The model under review builds one solid part; all positions refer to its coordinate system, in mm. Face numbers are marked on the shaded views. A direction names the side the tool comes from. Give positions to 0.01 mm unless a question says otherwise; leave off trailing zeros. Order: outer loops, then holes, each group sorted by start corner. A loop starts at its lowest first (then second) coordinate and runs counter-clockwise, first axis right, second up. Notation, with made-up numbers: (57, -29) - (68, -29) arc R21 ccw to (68, 7) - close; hole circle Ø3 at (49, 41). An arc over 180 degrees is marked (long way). Use CSV: the item, a comma, the result in double quotes. Start each with the question number.
1. Take a section at D-D, the plane x = 6. State the section outline as (y, z) points.
2. Take a section at B-B, the plane x = 43. State the section outline as (y, z) points.
3. Draft analysis for pull direction X (two halves, no side actions). For the marked faces 4, 5 and 6, state which applies: released by +X, released by -X, zero draft, split by the parting line, or undercut.
4. For pin 1 (6 mm diameter, centred on y = -4.5, z = -0.5, fed in from +X); pin 2 (2 mm diameter, centred on x = 15, y = -4.5, fed in from -Z); pin 3 (2 mm diameter, centred on y = -5, z = -4.5, fed in from -X), all flat-tipped, find the tip position at first contact; note any pin that passes through.
5. Take a section at A-A, the plane y = -3.25. State the section outline as (x, z) points.
6. Take a section at C-C, the plane y = 1.5. State the section outline as (x, z) points.
7. To check wall thickness, follow line 1 (Y direction, x = 36.5, z = -4.5); line 2 (X direction, y = 3, z = -2.25); line 3 (X direction, y = -1.75, z = -0.75). State the ranges of each line that lie inside material, in increasing order. Write a range as [from, to].
8. Machinability: for the marked faces 1, 2 and 3, which of the approach directions +Z, -Z, +X, -X, +Y, -Y give a long, thin tool a straight path to every point of the face, cutting with its end or side? Answer none if there is none.
```python
from build123d import *

# Parameters (mm, degrees)
BOSS_EXTRUDE1_DEPTH = 4
BOSS_EXTRUDE3_DEPTH = 2
BOSS_EXTRUDE4_DEPTH = 4
BOSS_EXTRUDE5_DEPTH = 2
BOSS_EXTRUDE6_DEPTH = 4


with BuildPart() as part:
    # Sketch1 → Boss-Extrude1 (new body)
    with BuildSketch(Plane(origin=(0, 0, 0), x_dir=(1, 0, 0), z_dir=(0, 1, 0))):
        with BuildLine():
            Line((-14.545827973, 6.554746402), (-17.81521366, 1.88557975))
            Line((-17.81521366, 1.88557975), (-10.442845262, -3.276608177))
            Line((-10.442845262, -3.276608177), (-8.148539516, -4))
            Line((-8.148539516, -4), (41.019227437, -1.767766953))
            Line((41.019227437, -1.767766953), (39.551460484, -0.3))
            Line((39.551460484, -0.3), (39.551460484, 4.117528082))
            ThreePointArc((39.551460484, 4.117528082), (40.137246921, 5.114213562), (41.133932401, 5.7))
            Line((41.133932401, 5.7), (47.010764551, 5.7))
            Line((47.010764551, 5.7), (47.251460484, 6))
            Line((47.251460484, 6), (47.251460484, 7))
            Line((47.251460484, 7), (27.251460484, 7))
            Line((27.251460484, 7), (27.251460484, 6))
            Line((27.251460484, 6), (25.251460484, 6))
            Line((25.251460484, 6), (25.251460484, 2))
            Line((25.251460484, 2), (16.751460484, 2))
            Line((16.751460484, 2), (16.751460484, 8.5))
            Line((16.751460484, 8.5), (-3.048539516, 8.5))
            Line((-3.048539516, 8.5), (-3.048539516, 2))
            Line((-3.048539516, 2), (-8.040975977, 2))
            Line((-8.040975977, 2), (-14.545827973, 6.554746402))
        make_face()
    extrude(amount=BOSS_EXTRUDE1_DEPTH)

    # Sketch1<7> → Boss-Extrude3 (add)
    with BuildSketch(Plane(origin=(0, 0, 0), x_dir=(1, 0, 0), z_dir=(0, 1, 0))):
        with BuildLine():
            ThreePointArc((10.010184156, 0.607136774), (5.101460484, 4.199275448), (0.192736812, 0.607136774))
            Line((0.192736812, 0.607136774), (0.192736812, -0.3))
            Line((0.192736812, -0.3), (-8.243129153, -0.3))
            Line((-8.243129153, -0.3), (-15.692980846, 4.916442314))
            Line((-15.692980846, 4.916442314), (-17.81521366, 1.88557975))
            Line((-17.81521366, 1.88557975), (-10.442845262, -3.276608177))
            Line((-10.442845262, -3.276608177), (-8.148539516, -4))
            Line((-8.148539516, -4), (41.019227437, -1.767766953))
            Line((41.019227437, -1.767766953), (39.551460484, -0.3))
            Line((39.551460484, -0.3), (39.251460484, -0.3))
            Line((39.251460484, -0.3), (39.051460484, -0.3))
            Line((39.051460484, -0.3), (10.010184156, -0.3))
            Line((10.010184156, -0.3), (10.010184156, 0.607136774))
        make_face()
    extrude(amount=-BOSS_EXTRUDE3_DEPTH)

    # Sketch1<8> → Boss-Extrude4 (add)
    with BuildSketch(Plane(origin=(0, 0, 0), x_dir=(1, 0, 0), z_dir=(0, 1, 0))):
        with BuildLine():
            Line((39.551460484, 0), (39.551460484, -0.3))
            Line((39.551460484, -0.3), (41.019227437, -1.767766953))
            Line((41.019227437, -1.767766953), (47.010764551, 5.7))
            Line((47.010764551, 5.7), (41.133932401, 5.7))
            ThreePointArc((41.133932401, 5.7), (40.598184056, 5.470750493), (40.137246921, 5.114213562))
            ThreePointArc((40.137246921, 5.114213562), (39.780709991, 4.653276427), (39.551460484, 4.117528082))
            Line((39.551460484, 4.117528082), (39.551460484, 0))
        make_face()
    extrude(amount=BOSS_EXTRUDE4_DEPTH)

    # Sketch1<9> → Boss-Extrude5 (add)
    with BuildSketch(Plane(origin=(0, 0, 0), x_dir=(1, 0, 0), z_dir=(0, 1, 0))):
        with BuildLine():
            Line((39.551460484, 0), (39.551460484, -0.3))
            Line((39.551460484, -0.3), (41.019227437, -1.767766953))
            Line((41.019227437, -1.767766953), (47.010764551, 5.7))
            Line((47.010764551, 5.7), (41.133932401, 5.7))
            ThreePointArc((41.133932401, 5.7), (40.598184056, 5.470750493), (40.137246921, 5.114213562))
            ThreePointArc((40.137246921, 5.114213562), (39.780709991, 4.653276427), (39.551460484, 4.117528082))
            Line((39.551460484, 4.117528082), (39.551460484, 0))
        make_face()
    extrude(amount=-BOSS_EXTRUDE5_DEPTH)

    # Sketch2 → Boss-Extrude6 (add)
    with BuildSketch(Plane(origin=(0, -2, 0), x_dir=(-1, 0, 0), z_dir=(0, -1, 0))):
        Polygon((-47.251460484, 7), (-47.251460484, 6), (-41.019227437, -1.767766953), (8.148539516, -4), (10.442845262, -3.276608177), (17.81521366, 1.88557975), (15.692980846, 4.916442314), (15.520907915, 5.162187927), (14.545827973, 6.554746402), (14.373755042, 6.800492016), (9.40586076, 3.32193499), (7.517941939, 2), (6.803867935, 1.5), (2.548539516, 1.5), (2.548539516, 7.5), (-16.751460484, 7.5), (-24.751460484, 7.5), (-24.751460484, 4.5), (-28.638302621, 4.5), (-33.251460484, 4.5), (-33.251460484, 7.5), (-37.214164404, 7.5), (-47.251460484, 7.5), align=None)
    extrude(amount=BOSS_EXTRUDE6_DEPTH)


solid = part.part
```
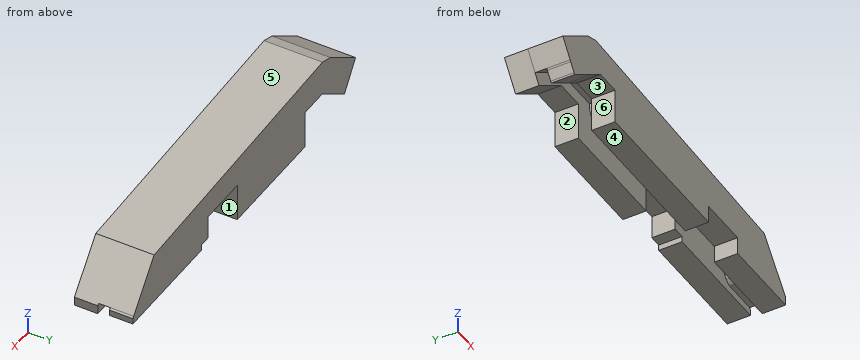
Determined:
1,outline,"(-6, -7.5) - (-2, -7.5) - (-2, -4.12) - (0, -4.12) - (0, -8.5) - (4, -8.5) - (4, 3.36) - (-6, 3.36) - close"
2,outline,"(-6, -7.5) - (-2, -7.5) - (-2, -5.7) - (0, -5.7) - (0, -7) - (4, -7) - (4, -0.7) - (-6, -0.7) - close"
3,face 4,"zero draft"
3,face 5,"released by +X"
3,face 6,"undercut"
4,pin 1,"stops at x = 45.25"
4,pin 2,"stops at z = -7.5"
4,pin 3,"stops at x = -16.68"
5,outline,"(-17.82, -1.89) - (-14.37, -6.8) - (-6.8, -1.5) - (-2.55, -1.5) - (-2.55, -7.5) - (24.75, -7.5) - (24.75, -4.5) - (33.25, -4.5) - (33.25, -7.5) - (47.25, -7.5) - (47.25, -6) - (41.02, 1.77) - (-8.15, 4) - (-10.44, 3.28) - close"
6,outline,"(-17.82, -1.89) - (-14.55, -6.55) - (-8.04, -2) - (-3.05, -2) - (-3.05, -8.5) - (16.75, -8.5) - (16.75, -2) - (25.25, -2) - (25.25, -6) - (27.25, -6) - (27.25, -7) - (47.25, -7) - (47.25, -6) - (41.02, 1.77) - (-8.15, 4) - (-10.44, 3.28) - close"
7,line 1,"y = [-6, -2], [0, 4]"
7,line 2,"x = [-17.56, -8.4], [-3.05, 16.75], [25.25, 44.24]"
7,line 3,"x = [-16.19, -9.74], [0.24, 9.96], [39.55, 43.04]"
8,face 1,"-Z, +Y"
8,face 2,"-Z, +Y, -Y"
8,face 3,"-Z, -Y"
